For this review, take the finished solid that the model builds, in its own axes (mm). A direction names the side the tool comes from. Give positions to 0.01 mm unless a question says otherwise; leave off trailing zeros. Order: outer loops, then holes, each group sorted by start corner. A loop starts at its lowest first (then second) coordinate and runs counter-clockwise, first axis right, second up. Notation, with made-up numbers: M 52,62.5 L 78,62.5 A28 cw 78,91.5 Z; hole C -27.75,-10.75 d6. An arc over 180 degrees is marked long. Answer as CSV lines item,"result". Start each with the question number.
1. For line 1 along Y through (x, z) = (25, 86.4); line 2 along Y through (x, z) = (45, 85.8); line 3 along Z through (x, y) = (-30, -11), list the stretches that pass through material, from the lowest coordinate up.
2. Clearance check with flat-ended pins moving along their axes: P1, Ø11, axis at y = -3, z = 65, coming from the -X side; P2, Ø25, axis at x = 36.5, y = -5.5, coming from the -Z side; P3, Ø6, axis at x = 25, y = -15, coming from the -Z side; P4, Ø4, axis at x = -12, z = 39, coming from the -Y side. State where each tip first meets the part, or that it passes through.
3. We need section B-B, the plane x = 0. Give the boundary of the cut face in (y, z).
4. Mouldability with a two-part tool opening along Z and no side actions: class faces 1 (the flat face through (1, 0, 87)), 2 (the cylindrical face through (23, -16.5, 85.5)), 3 (the flat face through (-5, 0, 64)), 4 (the cylindrical face through (-40, 0, -9)) as pulls with the +Z half, pulls with the -Z half, needs draft (parallel to the pull), parting line crosses it, or undercut.
5. We need section D-D, the plane z = 0. Give the boundary of the cut face in (x, y), and give its area (3 significant figures).
6. Machinability: for faces 5 (the flat face through (60, 0, 84)), 6 (the cylindrical face through (47.31, -0.96, 85.52)), 7 (the flat face through (5, 0, 64)), 8 (the flat face through (-33, 0, 82)), which of the approach directions +Z, -Z, +X, -X, +Y, -Y give a long, thin tool a straight path to every point of the face, cutting with its end or side? Answer none if there is none.
7. We need section A-A, the plane y = 0. Give the boundary of the cut face in (x, z).
8. We need section C-C, the plane y = 21.5. Give the boundary of the cut face in (x, z), and give its area (3 significant figures).
from build123d import *

# Parameters (mm, degrees)
SKETCH3_R           = 41
BOSS_EXTRUDE1_DEPTH = 24.75
SKETCH4_R           = 2.5
CUT_EXTRUDE1_DEPTH  = 30
CHAMFER1_SIZE       = 2


with BuildPart() as part:
    # Sketch3 → Boss-Extrude1 (new, symmetric)
    with BuildSketch(Plane(origin=(0, 0, 0), x_dir=(1, 0, 0), z_dir=(0, 1, 0))):
        with BuildLine():
            Line((5, -82), (60, -82))
            Line((60, -82), (60, -87))
            Line((60, -87), (-60, -87))
            Line((-60, -87), (-60, -82))
            Line((-60, -82), (-5, -82))
            Line((-5, -82), (-5, -45.727453461))
            ThreePointArc((-5, -45.727453461), (0, 46), (5, -45.727453461))
            Line((5, -45.727453461), (5, -82))
        make_face()
        with Locations(Location((0, 0, 0), (0, 0, 270))):
            Circle(SKETCH3_R, mode=Mode.SUBTRACT)
    extrude(amount=BOSS_EXTRUDE1_DEPTH, both=True)

    # Sketch4 → Cut-Extrude1 (cut)
    with BuildSketch(Plane.XY.offset(87)):
        with Locations((-25, 15)):
            Circle(SKETCH4_R)
        with Locations((-45, 0)):
            Circle(SKETCH4_R)
        with Locations((-25, -15)):
            Circle(SKETCH4_R)
        with Locations((25, -15)):
            Circle(SKETCH4_R)
        with Locations((45, 0)):
            Circle(SKETCH4_R)
        with Locations((25, 15)):
            Circle(SKETCH4_R)
    extrude(amount=-CUT_EXTRUDE1_DEPTH, mode=Mode.SUBTRACT)

    # Chamfer1
    chamfer1_edges = [part.edges().sort_by_distance(p)[0] for p in [
        (-47.5, 0, 82),
        (-27.5, 15, 82),
        (-27.5, -15, 82),
        (22.5, 15, 82),
        (22.5, -15, 82),
        (42.5, 0, 82),
    ]]
    chamfer(chamfer1_edges, length=CHAMFER1_SIZE)


solid = part.part
Result set:
1,line 1,"-24.75 to -17.5, -12.5 to 12.5, 17.5 to 24.75"
1,line 2,"-24.75 to -2.5, 2.5 to 24.75"
1,line 3,"-34.87 to -27.95, 27.95 to 34.87, 82 to 87"
2,P1,"x = -5"
2,P2,"z = -39.24"
2,P3,"z = -40.4"
2,P4,"y = -24.75"
3,outline,"M -24.75,-46 L 24.75,-46 L 24.75,-41 L -24.75,-41 Z; M -24.75,41 L 24.75,41 L 24.75,87 L -24.75,87 Z"
4,face 1,"pulls with the +Z half"
4,face 2,"needs draft"
4,face 3,"undercut"
4,face 4,"undercut"
5,outline,"M -46,-24.75 L -41,-24.75 L -41,24.75 L -46,24.75 Z; M 41,-24.75 L 46,-24.75 L 46,24.75 L 41,24.75 Z"
5,area,"495 mm2"
6,face 5,"+Z, -Z, +X, +Y, -Y"
6,face 6,"+Z"
6,face 7,"+X, +Y, -Y"
6,face 8,"-X, +Y, -Y"
7,outline,"M -60,82 L -49.5,82 L -47.5,84 L -47.5,87 L -60,87 Z; M -42.5,84 L -40.5,82 L -5,82 L -5,45.73 A46 ccw long 5,45.73 L 5,82 L 40.5,82 L 42.5,84 L 42.5,87 L -42.5,87 Z; M 47.5,84 L 49.5,82 L 60,82 L 60,87 L 47.5,87 Z; hole C 0,0 d82"
8,outline,"M -60,82 L -5,82 L -5,45.73 A46 ccw long 5,45.73 L 5,82 L 60,82 L 60,87 L -60,87 Z; hole C 0,0 d82"
8,area,"2,330 mm2"
